Check sheet for the modelled part. Datum: model origin and axes. Units: mm. Face numbers are marked on the shaded views. A direction names the side the tool comes from. Round coordinates to 2 decimals unless told otherwise and drop trailing zeros. Write each loop counter-clockwise with the first axis right and the second up, starting at its lowest first coordinate (ties: lowest second). Pieces come first, ordered by that corner, then holes. Notation, with made-up numbers: M 73,52 L 105,52 A15 ccw 105,76 Z; hole C 61.25,62 d4. An arc over 180 degrees is marked long. Put each result on its own line as item: value.
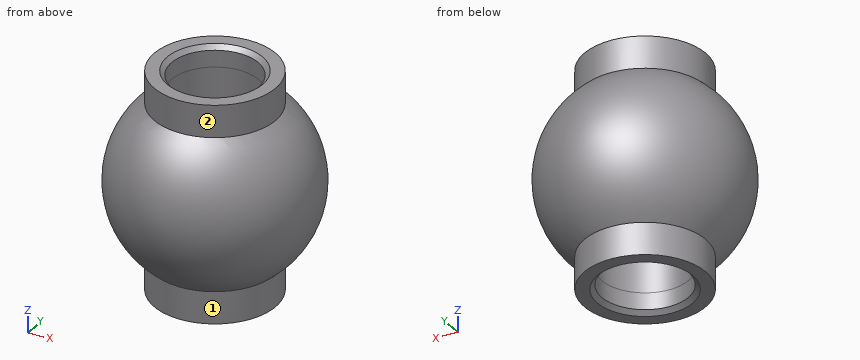
```python
from build123d import *

# Parameters (mm, degrees)
CUT_EXTRUDE4_DEPTH      = 45.534963442
CUT_EXTRUDE4_DEPTH_BACK = 45.534963442
SKETCH10_R              = 6.35
SKETCH12_R              = 8.89
SKETCH12_R_2            = 6.35
EXTRUDE1_DEPTH          = 15.875
CHAMFER1_SIZE           = 0.635


with BuildPart() as part:
    # Sketch7 → Revolve3 (revolve)
    with BuildSketch(Plane.XY):
        with BuildLine():
            Line((0, 39.6875), (0, 11.1125))
            ThreePointArc((0, 11.1125), (14.2875, 25.4), (0, 39.6875))
        make_face()
    revolve(axis=Axis((0, 0, 0), (0, 1, 0)))

    # Sketch10 → Cut-Extrude4 (cut, two sides: drawn at the far end of the back side and taken through both)
    with BuildSketch(Plane.XY.offset(-CUT_EXTRUDE4_DEPTH_BACK)):
        with Locations((0, 25.4)):
            Circle(SKETCH10_R)
    extrude(amount=CUT_EXTRUDE4_DEPTH + CUT_EXTRUDE4_DEPTH_BACK, mode=Mode.SUBTRACT)

    # Sketch12 → Extrude1 (add, symmetric)
    with BuildSketch(Plane.XY):
        with Locations(Location((0, 25.4, 0), (0, 0, 180))):
            Circle(SKETCH12_R)
        with Locations((0, 25.4)):
            Circle(SKETCH12_R_2, mode=Mode.SUBTRACT)
    extrude(amount=EXTRUDE1_DEPTH, both=True)

    # Chamfer1
    chamfer1_edges = [part.edges().sort_by_distance(p)[0] for p in [
        (-6.35, 25.4, -15.875),
        (-6.35, 25.4, 15.875),
    ]]
    chamfer(chamfer1_edges, length=CHAMFER1_SIZE)


solid = part.part
```
1. Cross-section at C-C (z = 13.5). Enter the section's corners in (x, y).
Computed values:
outline: C 0,25.4 d17.78; hole C 0,25.4 d12.7
2. Scan lines: probe 1 along Y at (x, z) = (0, 13.6); probe 2 along X at (y, z) = (25.4, -14.3); probe 3 along X at (y, z) = (25.4, 0). Record each from-to range of solid material in increasing order.
Computed values:
probe 1: y = 16.51 to 19.05, 31.75 to 34.29
probe 2: x = -8.89 to -6.35, 6.35 to 8.89
probe 3: x = -14.29 to -6.35, 6.35 to 14.29
3. Depth check by flat-ended pin: pin 1 Ø4 at (y, z) = (23.5, -3) entering from -X; pin 2 Ø4 at (y, z) = (27.5, -3) entering from +X; pin 3 Ø12 at (x, z) = (5, 6.5) entering from -Y; pin 4 Ø7.5 at (x, y) = (0, 25.4) entering from +Z. Enter the tip coordinate at first touch or a pass-through.
Computed values:
pin 1: stops at x = -14.2
pin 2: stops at x = 14.19
pin 3: stops at y = 11.28
pin 4: passes through
4. Cross-section at D-D (x = 11.5). Enter the section's corners in (y, z).
Computed values:
outline: C 25.4,0 d16.96
5. Access from +Z, -Z, +X, -X, +Y, -Y to the whole of each face (thin tool, end or side, straight path). Record for the marked faces 1 and 2.
Computed values:
face 1: -Z
face 2: +Z
